from build123d import *

# Parameters (mm, degrees)
F0_W     = 50.8
F0_H     = 12.7
F1_DEPTH = 50.8
F2_DEPTH = 12.7
F3_R     = 6.35
F4_DEPTH = 12.7
F5_R     = 6.35
F6_DEPTH = 12.7


with BuildPart() as f1:
    # F0 (on Front) → F1 (new body)
    with BuildSketch(Plane.XZ):
        with Locations((0, 6.35)):
            Rectangle(F0_W, F0_H)
    extrude(amount=F1_DEPTH)



with BuildPart() as f1b:
    # F0 (on Front) → F1, piece 2 (new body)
    with BuildSketch(Plane.XZ):
        Polygon((-50.8, 165.1), (-53.2678634281, 152.6420848413), (-0.3815758649, 142.1655216876), (2.0862875631, 154.6234368462), align=None)
    extrude(amount=F1_DEPTH)


with BuildPart() as f1_1:
    add(f1.part)

    add(f1b.part)  # F2 merges F1b
    # F0 (on Front) → F2 (join)
    with BuildSketch(Plane.XZ):
        Polygon((-53.2678634281, 152.6420848413), (-25.4, 12.7), (25.4, 12.7), (-0.3815758649, 142.1655216876), align=None)
    extrude(amount=F2_DEPTH)

    # F3 (on face) → F4 (cut, through all)
    with BuildSketch(Plane(origin=(0, 0, 0), x_dir=(1, 0, 0), z_dir=(0, 0, -1))):
        with Locations((0, 33.3375)):
            Circle(F3_R)
    extrude(amount=-F4_DEPTH, mode=Mode.SUBTRACT)

    # F5 (on face) → F6 (cut, through all)
    with BuildSketch(Plane(origin=(29.5524592231, 0, 149.1824975169), x_dir=(0.9809382015, 0, -0.194319955), z_dir=(0.194319955, 0, 0.9809382015))):
        with Locations((-56.5138851996, -33.3375)):
            Circle(F5_R)
    extrude(amount=-F6_DEPTH, mode=Mode.SUBTRACT)


solid = f1_1.part
Read the model definition and answer for the solid it produces. Units are mm, in the model's axes. A direction names the side the tool comes from. Give positions to 0.01 mm unless a question says otherwise; leave off trailing zeros. Write each loop counter-clockwise with the first axis right and the second up, starting at its lowest first coordinate (ties: lowest second). Pieces come first, ordered by that corner, then holes. Notation, with made-up numbers: (-1, -21.75) - (57, -21.75) arc R21 ccw to (57, -8.75) - close; hole circle Ø10 at (51.5, 8.5). An arc over 180 degrees is marked (long way). Return JSON: item names as keys, results as strings.
Q1. A cutting plane is placed at C-C, the plane x = -10. Determine the outline of the cut face in (y, z), and give its area (3 significant figures).
Reply:
{"outline": "(-50.8, 0) - (0, 0) - (0, 157.02) - (-50.8, 157.02) - (-50.8, 144.07) - (-12.7, 144.07) - (-12.7, 12.7) - (-50.8, 12.7) - close", "area": "2,970 mm²"}
Q2. Consider line 1 along Y through (x, z) = (0, 5.75); line 2 along Y through (x, z) = (-8.5, 100); line 3 along Z through (x, y) = (-6, -17). Determine where each line is inside the solid, lowest interval first. Write a range as [from, to].
Reply:
{"line 1": "[-50.8, -39.69], [-26.99, 0]", "line 2": "[-12.7, 0]", "line 3": "[0, 12.7], [143.28, 156.23]"}
Q3. Given P1, Ø12, axis at x = -18, y = -43.5, coming from the -Z side; P2, Ø4, axis at x = -40, z = 138.5, coming from the -Y side; P3, Ø11.5, axis at x = 11.5, y = -28, coming from the +Z side; P4, Ø5, axis at y = -7.5, z = 138, coming from the +X side, each flat-ended and moving along its own axis, determine where each tip first touches the part or whether it passes through.
Reply:
{"P1": "z = 0", "P2": "y = -12.7", "P3": "z = 12.7", "P4": "x = 0.95"}
Q4. For faces 4 (the face through (-21.319, -31.483, 146.313)), 5 (the face through (0.835, -25.044, 148.307)), 6 (the face through (2.93, -27.704, 6.261)), determine the directions among +Z, -Z, +X, -X, +Y, -Y from which every point of the face is accessible in a straight line to the end or side of a thin tool.
Reply:
{"face 4": "-X, -Y", "face 5": "+X, +Y, -Y", "face 6": "-Z"}
Q5. A cutting plane is placed at A-A, the plane y = -47. Determine the outline of the cut face in (x, z).
Reply:
{"outline": "(-53.27, 152.64) - (-0.38, 142.17) - (2.09, 154.62) - (-50.8, 165.1) - close; (-25.4, 0) - (25.4, 0) - (25.4, 12.7) - (-25.4, 12.7) - close"}
Q6. A cutting plane is placed at B-B, the plane x = -44. Determine the outline of the cut face in (y, z).
Reply:
{"outline": "(-50.8, 150.81) - (-12.7, 150.81) - (-12.7, 106.1) - (0, 106.1) - (0, 163.75) - (-50.8, 163.75) - close"}
Q7. For a pull along X with two mould halves and no side action, classify faces 1 (the face through (-14, 0, 84)), 2 (the face through (-25.4, -25, 6)), 3 (the face through (-24.227, -38.971, 153.453)) as released by +X, released by -X, zero draft, split by the parting line, or undercut.
Reply:
{"face 1": "zero draft", "face 2": "released by -X", "face 3": "undercut"}
Q8. A cutting plane is placed at D-D, the plane z = 69.5. Determine the outline of the cut face in (x, y).
Reply:
{"outline": "(-36.71, -12.7) - (14.09, -12.7) - (14.09, 0) - (-36.71, 0) - close"}
